from build123d import *

# Parameters (mm, degrees)
BOSS_EXTRUDE1_DEPTH = 254


with BuildPart() as part:
    # Sketch1 → Boss-Extrude1 (new body)
    with BuildSketch(Plane.XY):
        with BuildLine():
            Line((0, 0), (190.632291842, 0))
            Line((190.632291842, 0), (190.632291842, 76.2))
            Line((190.632291842, 76.2), (63.745532682, 76.2))
            ThreePointArc((63.745532682, 76.2), (-126.867708158, 208.995224478), (-317.480948998, 76.2))
            Line((-317.480948998, 76.2), (-444.367708158, 76.2))
            Line((-444.367708158, 76.2), (-444.367708158, 0))
            Line((-444.367708158, 0), (-253.735416316, 0))
            ThreePointArc((-253.735416316, 0), (-126.867708158, 132.795224478), (0, 0))
        make_face()
    extrude(amount=-BOSS_EXTRUDE1_DEPTH)


solid = part.part
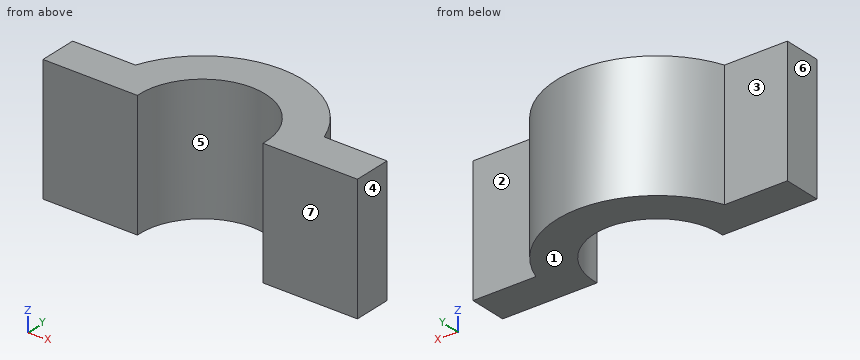
Here's how the part is built. I have some questions about the finished solid (model axes, mm). Face numbers are marked on the shaded views. A direction names the side the tool comes from. Coordinates: 2 decimals unless noted, no trailing zeros. Write each loop counter-clockwise with the first axis right and the second up, starting at its lowest first coordinate (ties: lowest second). Pieces come first, ordered by that corner, then holes.
1) Thinking about a two-plate mould opening in X: for the marked faces 4, 5, 6 and 7, which applies, +X half, -X half, draft (parallel to the pull), parting line (faces both ways), or undercut?
Filled in:
face 4: +X half
face 5: undercut
face 6: -X half
face 7: draft
2) If we section it at D-D (y = 34): List the corners of the cut face in (x, z) for me.
Filled in:
outline: (-444.37, -254) - (-250.7, -254) - (-250.7, 0) - (-444.37, 0) - close; (-3.04, -254) - (190.63, -254) - (190.63, 0) - (-3.04, 0) - close
3) If we section it at C-C (x = -368.5): List the corners of the cut face in (y, z) for me, plus the area to 3 significant figures.
Filled in:
outline: (0, -254) - (76.2, -254) - (76.2, 0) - (0, 0) - close
area: 19,400 mm2
4) If I drill on line 1 (X direction, y = 11, z = -180); line 2 (Y direction, x = 70, z = -229.5); line 3 (X direction, y = 76, z = -66.5), over which ranges is the centre line in solid material (lowest first)?
Filled in:
line 1: x = -444.37 to -253.76, 0.03 to 190.63
line 2: y = 0 to 76.2
line 3: x = -444.37 to -232.7, -21.04 to 190.63
5) If we section it at B-B (z = -75): List the corners of the cut face in (x, y) for me, plus the area to 3 significant figures.
Filled in:
outline: (-444.37, 0) - (-253.74, 0) arc R127 cw (long way) to (0, 0) - (190.63, 0) - (190.63, 76.2) - (63.75, 76.2) arc R203.2 ccw to (-317.48, 76.2) - (-444.37, 76.2) - close
area: 58,400 mm2
6) If we section it at A-A (y = 120.5): List the corners of the cut face in (x, z) for me.
Filled in:
outline: (-294.6, -254) - (-181.38, -254) - (-181.38, 0) - (-294.6, 0) - close; (-72.35, -254) - (40.86, -254) - (40.86, 0) - (-72.35, 0) - close
7) Which directions (+Z, -Z, +X, -X, +Y, -Y) give clear straight access to the entire face, cutting with the end or side of a thin tool? Please do the marked faces 1, 2 and 3.
Filled in:
face 1: -Z, +X, -X, +Y, -Y
face 2: +Z, -Z, +X, +Y
face 3: +Z, -Z, -X, +Y
8) I'm going to push flat-ended pins straight in: pin 1 (3 mm diameter, centred on y = 122, z = -52.5, fed in from -X); pin 2 (1 mm diameter, centred on x = -85, z = -30.5, fed in from +Y); pin 3 (6 mm diameter, centred on y = 115, z = -220, fed in from +X). Where does each tip first touch, or does it pass through?
Filled in:
pin 1: stops at x = -294.6
pin 2: stops at y = 204.74
pin 3: stops at x = 46.37
